Geometry check sheet. Reference: drawing and pictorial views, mm from the part's lowest x, y, z. A direction names the side the tool comes from. Coordinates: 2 decimals unless noted, no trailing zeros. Write each loop counter-clockwise with the first axis right and the second up, starting at its lowest first coordinate (ties: lowest second). Pieces come first, ordered by that corner, then holes. Notation, with made-up numbers: M -23,-17.75 L 9,-17.75 A36 cw 9,17.25 Z; hole C 1.5,-20.5 d11. An arc over 180 degrees is marked long. One line per item, written item: value.
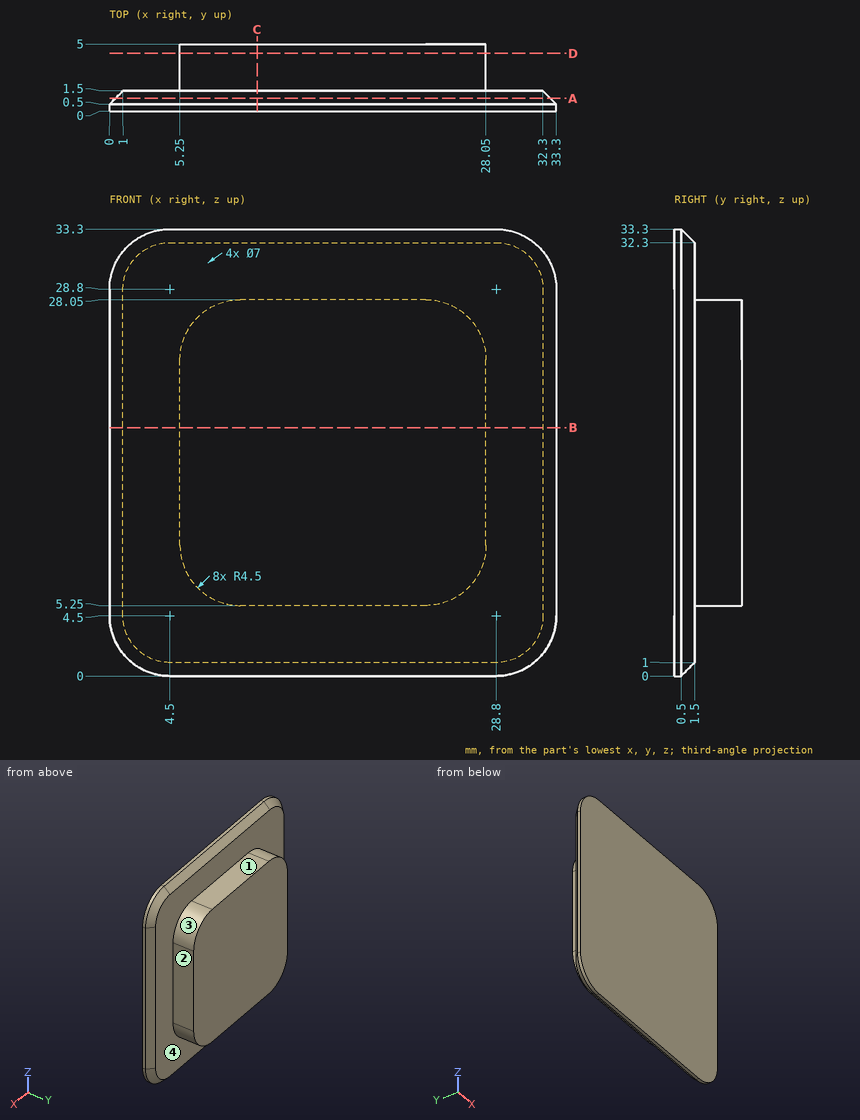
Item 1: Cross-section at B-B, the plane z = 18.5. Enter the section's corners in (x, y), and give its area (3 significant figures).
The answers:
outline: M 0,0 L 33.3,0 L 33.3,0.5 L 32.3,1.5 L 28.05,1.5 L 28.05,5 L 5.25,5 L 5.25,1.5 L 1,1.5 L 0,0.5 Z
area: 129 mm²
Item 2: Scan lines: line 1 (Z direction, x = 21.5, y = 3.3); line 2 (Y direction, x = 4.5, z = 25). Record each from-to range of solid material in increasing order.
The answers:
line 1: z = 5.25 to 28.05
line 2: y = 0 to 1.5
Item 3: Go/stop test with flat-tipped pins: P1, Ø1.5, axis at x = 11.5, z = 15.5, coming from the -Y side; P2, Ø1.5, axis at y = 2, z = 23.5, coming from the +X side; P3, Ø1.5, axis at y = 2, z = 27.5, coming from the -X side; P4, Ø1, axis at y = 3, z = 13.5, coming from the -X side. Record where each tip stops, or that it passes through.
The answers:
P1: stops at y = 0
P2: stops at x = 32.55
P3: stops at x = 0.75
P4: stops at x = 5.25
Item 4: Cross-section at A-A, the plane y = 0.95. Enter the section's corners in (x, z), and give its area (3 significant figures).
The answers:
outline: M 0.45,4.5 A4.05 ccw 4.5,0.45 L 28.8,0.45 A4.05 ccw 32.85,4.5 L 32.85,28.8 A4.05 ccw 28.8,32.85 L 4.5,32.85 A4.05 ccw 0.45,28.8 Z
area: 1,040 mm²
Item 5: Cross-section at D-D, the plane y = 4.3. Enter the section's corners in (x, z).
The answers:
outline: M 5.25,9.75 A4.5 ccw 9.75,5.25 L 23.55,5.25 A4.5 ccw 28.05,9.75 L 28.05,23.55 A4.5 ccw 23.55,28.05 L 9.75,28.05 A4.5 ccw 5.25,23.55 Z
Item 6: Access from +Z, -Z, +X, -X, +Y, -Y to the whole of each face (thin tool, end or side, straight path). Record for the marked faces 1, 2, 3 and 4.
The answers:
face 1: +Z, +X, -X, +Y
face 2: +Z, -Z, +X, +Y
face 3: +Z, +X, +Y
face 4: +Y
Item 7: Cross-section at C-C, the plane x = 11. Enter the section's corners in (y, z), and give its area (3 significant figures).
The answers:
outline: M 0,0 L 0.5,0 L 1.5,1 L 1.5,5.25 L 5,5.25 L 5,28.05 L 1.5,28.05 L 1.5,32.3 L 0.5,33.3 L 0,33.3 Z
area: 129 mm²
